from build123d import *

# Parameters (mm, degrees)
F1_DEPTH        = 25
F3_DEPTH        = 25.001
F3_COPIES_COUNT = 10
F4_R            = 25
F5_DEPTH        = 25.001
F6_R            = 15
F7_DEPTH        = 25.001
F7_COPIES_COUNT = 6


# Not quite as in the source:
# - a pattern or mirror of a feature is missing from the dataset's text; its kind, count and spacing are read off the source's solid


with BuildPart() as f1:
    # F0 (on Front) → F1 (new body)
    with BuildSketch(Plane.XZ):
        with BuildLine():
            Line((-8.9100863455, 98.6570205686), (0, 100))
            Line((0, 100), (13.2558165823, 98.002007127))
            Line((13.2558165823, 98.002007127), (20.2559942473, 104.8591660301))
            ThreePointArc((20.2559942473, 104.8591660301), (22.9030212669, 107.1136465319), (25.8372403083, 108.979066858))
            ThreePointArc((25.8372403083, 108.979066858), (0, 112), (-25.8372403083, 108.979066858))
            ThreePointArc((-25.8372403083, 108.979066858), (-22.9030212669, 107.1136465319), (-20.2559942473, 104.8591660301))
            Line((-20.2559942473, 104.8591660301), (-13.2558165823, 98.002007127))
            Line((-13.2558165823, 98.002007127), (-8.9100863455, 98.6570205686))
        make_face()
        with BuildLine():
            Line((20.2559942473, 104.8591660301), (13.2558165823, 98.002007127))
            Line((13.2558165823, 98.002007127), (29.4755174411, 95.5572805786))
            Line((29.4755174411, 95.5572805786), (56.3320058064, 82.6238774316))
            Line((56.3320058064, 82.6238774316), (78.1831482468, 62.3489801859))
            Line((78.1831482468, 62.3489801859), (93.0873748644, 36.5341024366))
            Line((93.0873748644, 36.5341024366), (99.7203797181, 7.4730093586))
            Line((99.7203797181, 7.4730093586), (97.4927912182, -22.2520933956))
            Line((97.4927912182, -22.2520933956), (86.6025403784, -50))
            Line((86.6025403784, -50), (68.0172737771, -73.305187183))
            Line((68.0172737771, -73.305187183), (43.3883739118, -90.0968867902))
            Line((43.3883739118, -90.0968867902), (14.9042266176, -98.8830826225))
            Line((14.9042266176, -98.8830826225), (-14.9042266176, -98.8830826225))
            Line((-14.9042266176, -98.8830826225), (-43.3883739118, -90.0968867902))
            Line((-43.3883739118, -90.0968867902), (-68.0172737771, -73.305187183))
            Line((-68.0172737771, -73.305187183), (-86.6025403784, -50))
            Line((-86.6025403784, -50), (-97.4927912182, -22.2520933956))
            Line((-97.4927912182, -22.2520933956), (-99.7203797181, 7.4730093586))
            Line((-99.7203797181, 7.4730093586), (-93.0873748644, 36.5341024366))
            Line((-93.0873748644, 36.5341024366), (-78.1831482468, 62.3489801859))
            Line((-78.1831482468, 62.3489801859), (-56.3320058064, 82.6238774316))
            Line((-56.3320058064, 82.6238774316), (-29.4755174411, 95.5572805786))
            Line((-29.4755174411, 95.5572805786), (-13.2558165823, 98.002007127))
            Line((-13.2558165823, 98.002007127), (-20.2559942473, 104.8591660301))
            ThreePointArc((-20.2559942473, 104.8591660301), (-22.9030212669, 107.1136465319), (-25.8372403083, 108.979066858))
            ThreePointArc((-25.8372403083, 108.979066858), (-69.463044439, -87.857187852), (112, 0))
            ThreePointArc((112, 0), (87.857187852, 69.463044439), (25.8372403083, 108.979066858))
            ThreePointArc((25.8372403083, 108.979066858), (22.9030212669, 107.1136465319), (20.2559942473, 104.8591660301))
        make_face()
        with BuildLine():
            ThreePointArc((90, 0), (63.957016816, 63.3206127576), (0.9, 89.9954998875))
            ThreePointArc((0.9, 89.9954998875), (0, 90), (-0.9, 89.9954998875))
            ThreePointArc((-0.9, 89.9954998875), (-63.3206127576, -63.957016816), (90, 0))
        make_face()
        with BuildLine():
            Line((29.4755174411, 95.5572805786), (13.2558165823, 98.002007127))
            Line((13.2558165823, 98.002007127), (7.9977160698, 92.851333463))
            ThreePointArc((7.9977160698, 92.851333463), (4.7327694943, 90.7178003028), (0.9, 89.9954998875))
            ThreePointArc((0.9, 89.9954998875), (63.957016816, 63.3206127576), (90, 0))
            ThreePointArc((90, 0), (-63.3206127576, -63.957016816), (-0.9, 89.9954998875))
            ThreePointArc((-0.9, 89.9954998875), (-4.7327694943, 90.7178003028), (-7.9977160698, 92.851333463))
            Line((-7.9977160698, 92.851333463), (-13.2558165823, 98.002007127))
            Line((-13.2558165823, 98.002007127), (-29.4755174411, 95.5572805786))
            Line((-29.4755174411, 95.5572805786), (-56.3320058064, 82.6238774316))
            Line((-56.3320058064, 82.6238774316), (-78.1831482468, 62.3489801859))
            Line((-78.1831482468, 62.3489801859), (-93.0873748644, 36.5341024366))
            Line((-93.0873748644, 36.5341024366), (-99.7203797181, 7.4730093586))
            Line((-99.7203797181, 7.4730093586), (-97.4927912182, -22.2520933956))
            Line((-97.4927912182, -22.2520933956), (-86.6025403784, -50))
            Line((-86.6025403784, -50), (-68.0172737771, -73.305187183))
            Line((-68.0172737771, -73.305187183), (-43.3883739118, -90.0968867902))
            Line((-43.3883739118, -90.0968867902), (-14.9042266176, -98.8830826225))
            Line((-14.9042266176, -98.8830826225), (14.9042266176, -98.8830826225))
            Line((14.9042266176, -98.8830826225), (43.3883739118, -90.0968867902))
            Line((43.3883739118, -90.0968867902), (68.0172737771, -73.305187183))
            Line((68.0172737771, -73.305187183), (86.6025403784, -50))
            Line((86.6025403784, -50), (97.4927912182, -22.2520933956))
            Line((97.4927912182, -22.2520933956), (99.7203797181, 7.4730093586))
            Line((99.7203797181, 7.4730093586), (93.0873748644, 36.5341024366))
            Line((93.0873748644, 36.5341024366), (78.1831482468, 62.3489801859))
            Line((78.1831482468, 62.3489801859), (56.3320058064, 82.6238774316))
            Line((56.3320058064, 82.6238774316), (29.4755174411, 95.5572805786))
        make_face()
        with BuildLine():
            Line((13.2558165823, 98.002007127), (0, 100))
            Line((0, 100), (-8.9100863455, 98.6570205686))
            Line((-8.9100863455, 98.6570205686), (-13.2558165823, 98.002007127))
            Line((-13.2558165823, 98.002007127), (-7.9977160698, 92.851333463))
            ThreePointArc((-7.9977160698, 92.851333463), (-4.7327694943, 90.7178003028), (-0.9, 89.9954998875))
            ThreePointArc((-0.9, 89.9954998875), (0, 90), (0.9, 89.9954998875))
            ThreePointArc((0.9, 89.9954998875), (4.7327694943, 90.7178003028), (7.9977160698, 92.851333463))
            Line((7.9977160698, 92.851333463), (13.2558165823, 98.002007127))
        make_face()
    extrude(amount=F1_DEPTH)

    # F2 (on face) → F3 (cut, through all)
    with BuildSketch(Plane.XZ.offset(25)):
        with BuildLine():
            ThreePointArc((-25.8372403083, 108.979066858), (-22.9030212669, 107.1136465319), (-20.2559942473, 104.8591660301))
            Line((-20.2559942473, 104.8591660301), (-7.9977160698, 92.851333463))
            ThreePointArc((-7.9977160698, 92.851333463), (-4.7327694943, 90.7178003028), (-0.9, 89.9954998875))
            ThreePointArc((-0.9, 89.9954998875), (0, 90), (0.9, 89.9954998875))
            ThreePointArc((0.9, 89.9954998875), (4.7327694943, 90.7178003028), (7.9977160698, 92.851333463))
            Line((7.9977160698, 92.851333463), (20.2559942473, 104.8591660301))
            ThreePointArc((20.2559942473, 104.8591660301), (22.9030212669, 107.1136465319), (25.8372403083, 108.979066858))
            ThreePointArc((25.8372403083, 108.979066858), (0, 112), (-25.8372403083, 108.979066858))
        make_face()
    f3 = extrude(amount=-F3_DEPTH, mode=Mode.SUBTRACT)

    # F3_copies: F3 ×10 about axis
    f3_copies_axis = Axis((0, 0, 0), (0, 1, 0))
    for i in range(1, F3_COPIES_COUNT):
        add(f3.rotate(f3_copies_axis, i * 360 / F3_COPIES_COUNT), mode=Mode.SUBTRACT)

    # F4 (on face) → F5 (cut, through all)
    with BuildSketch(Plane.XZ.offset(25)):
        Circle(F4_R)
    extrude(amount=-F5_DEPTH, mode=Mode.SUBTRACT)

    # F6 (on face) → F7 (cut, through all)
    with BuildSketch(Plane.XZ.offset(25)):
        with Locations((0, 56.8999728613)):
            Circle(F6_R)
    f7 = extrude(amount=-F7_DEPTH, mode=Mode.SUBTRACT)

    # F7_copies: F7 ×6 about axis
    f7_copies_axis = Axis((0, 0, 0), (0, 1, 0))
    for i in range(1, F7_COPIES_COUNT):
        add(f7.rotate(f7_copies_axis, i * 360 / F7_COPIES_COUNT), mode=Mode.SUBTRACT)


solid = f1.part
The listing builds one solid part. Answer for the finished solid, in the listing's coordinates (mm). A direction names the side the tool comes from. Coordinates: 2 decimals unless noted, no trailing zeros. Loops run counter-clockwise (first coordinate to the right, second up) from the corner with the lowest first, then second, coordinate; pieces in that order, holes last. Notation, with made-up numbers: (86, -23) -> (141, -23) arc R29 ccw to (141, -1) -> close; hole circle Ø10 at (69.25, 65). An arc over 180 degrees is marked (long way). Answer in a Markdown table with one row per item. Add a question column.
1. The part is cut by section A-A, the plane z = 0. Write down the section's boundary in (x, y), then the cut area to 3 significant figures.
2. Flat-ended cylindrical pins translate along their axes: P1, Ø4, axis at y = -14.5, z = 85, coming from the +X side; P2, Ø1.5, axis at x = -13.5, y = -16.5, coming from the -Z side; P3, Ø5, axis at x = -10.5, y = -18.5, coming from the -Z side. Find the tip coordinate at first contact, or state that the pin passes through.
3. The part is cut by section B-B, the plane y = -12.5. Count the separate pieces of the cut face and the enclosed holes in it, then the cut area to 3 significant figures.
4. Determine the mould class of faces 3 (the flat face through (98.276, -12.675, 17.168)), 4 (the cylindrical face through (-4.682, -12.675, -90.697)), 5 (the cylindrical face through (-22.86, -12.68, -107.08)), 6 (the cylindrical face through (-84.81, -12.68, 32.48)) for opening direction X: +X half, -X half, draft (parallel to the pull), parting line (faces both ways), or undercut.
5. Consider line 1 (Z direction, x = 0, y = -14.5); line 2 (X direction, y = -19.75, z = -0.5) (3 decimals); line 3 (X direction, y = -6, z = 16.5). Determine where each line is inside the solid, lowest interval first. Write a range as [from, to].
6. For faces 1 (the flat face through (-46.697, -12.675, 88.161)), 2 (the flat face through (98.489, -12.675, -17.057)), determine the directions among +Z, -Z, +X, -X, +Y, -Y from which every point of the face is accessible in a straight line to the end or side of a thin tool.
Answer below:
| question | item | result |
|---|---|---|
| 1 | outline | (-112, -25) -> (-25, -25) -> (-25, 0) -> (-112, 0) -> close; (25, -25) -> (112, -25) -> (112, 0) -> (25, 0) -> close |
| 1 | area | 4,350 mm2 |
| 2 | P1 | x = 47.57 |
| 2 | P2 | z = -98.98 |
| 2 | P3 | z = -97.75 |
| 3 | separate pieces | 1 |
| 3 | enclosed holes | 7 |
| 3 | area | 26,600 mm2 |
| 4 | face 3 | +X half |
| 4 | face 4 | undercut |
| 4 | face 5 | undercut |
| 4 | face 6 | -X half |
| 5 | line 1 | [-90, -71.9], [-41.9, -25], [25, 41.9], [71.9, 90] |
| 5 | line 2 | [-111.999, -24.995], [24.995, 111.999] |
| 5 | line 3 | [-99.55, -58.34], [-40.21, -18.78], [18.78, 40.21], [58.34, 99.55] |
| 6 | face 1 | +Z, -X, +Y, -Y |
| 6 | face 2 | +X, +Y, -Y |
